```python
from build123d import *

# Parameters (mm, degrees)
EXTRUDE_1_DEPTH     = 10
SKETCH_4_R          = 1.6
CUT_EXTRUDE_1_DEPTH = 10


with BuildPart() as part:
    # 草图3 → 凸台-拉伸1 (new body)
    with BuildSketch(Plane(origin=(0, 0, 0), x_dir=(0, 0, -1), z_dir=(0.7071067811865488, 0.7071067811865464, 0))):
        with BuildLine():
            Line((0, 2), (0, 9))
            Line((0, 9), (-4, 9))
            Line((-4, 9), (-4, -9))
            Line((-4, -9), (0, -9))
            Line((0, -9), (0, -2))
            ThreePointArc((0, -2), (-2, 0), (0, 2))
        make_face()
    extrude(amount=EXTRUDE_1_DEPTH)

    # 草图4 → 切除-拉伸1 (cut)
    with BuildSketch(Plane.XY.offset(4)):
        with Locations((0, 8)):
            Circle(SKETCH_4_R)
        with Locations((8, 0)):
            Circle(SKETCH_4_R)
    extrude(amount=-CUT_EXTRUDE_1_DEPTH, mode=Mode.SUBTRACT)


solid = part.part
```
Verification items for the finished model (mm, model axes). Give positions to 0.01 mm unless a question says otherwise; leave off trailing zeros. Write each loop counter-clockwise with the first axis right and the second up, starting at its lowest first coordinate (ties: lowest second). Pieces come first, ordered by that corner, then holes. Notation, with made-up numbers: (89, 84) - (121, 84) arc R14 ccw to (121, 91) - close; hole circle Ø5 at (-35.5, 82.25). An arc over 180 degrees is marked (long way). Put each result on its own line as item: value.
Q1. Section check C-C on y = -3.75. Record the cut outline in (x, z).
Result:
outline: (3.75, 0) - (8.98, 0) - (8.98, 4) - (3.75, 4) - close
Q2. Section check A-A on z = 0.55. Record the cut outline in (x, y).
Result:
outline: (-6.36, 6.36) - (-1.36, 1.36) - (5.71, 8.43) - (0.71, 13.44) - close; (1.36, -1.36) - (6.36, -6.36) - (13.44, 0.71) - (8.43, 5.71) - close; hole circle Ø3.2 at (0, 8); hole circle Ø3.2 at (8, 0)
Q3. Section check B-B on z = 3.4. Record the cut outline in (x, y), and give its area (3 significant figures).
Result:
outline: (-6.36, 6.36) - (6.36, -6.36) - (13.44, 0.71) - (0.71, 13.44) - close; hole circle Ø3.2 at (0, 8); hole circle Ø3.2 at (8, 0)
area: 164 mm2
Q4. Mould release check, pull along Y, two halves, no side actions. Record for faces 1 (the face through (6.4, 0.07, 2.03)), 2 (the face through (-0.35, 6.44, 2.03)), 3 (the face through (-2.88, 9.85, 1.97)), 4 (the face through (-0.1, 0.1, 2.5)): released by +Y, released by -Y, zero draft, split by the parting line, or undercut.
Result:
face 1: undercut
face 2: undercut
face 3: released by +Y
face 4: released by -Y
Q5. Scan lines: probe 1 along Y at (x, z) = (8, 2.75); probe 2 along X at (y, z) = (4.5, 1.35); probe 3 along Y at (x, z) = (0, 2.85). Record each from-to range of solid material in increasing order. Write a range as from..to.
Result:
probe 1: -4.73..-1.6, 1.6..6.14
probe 2: -4.5..2.41, 6.59..9.64
probe 3: 0..6.4, 9.6..12.73
Q6. Depth check by flat-ended pin: P1, Ø1.9, axis at x = 0, y = 8, coming from the +Z side; P2, Ø1.5, axis at y = 11, z = 1.5, coming from the -X side; P3, Ø1, axis at y = 2.5, z = 2.5, coming from the +X side. Enter the tip coordinate at first touch or a pass-through.
Result:
P1: through
P2: x = -2.48
P3: x = 12.14
